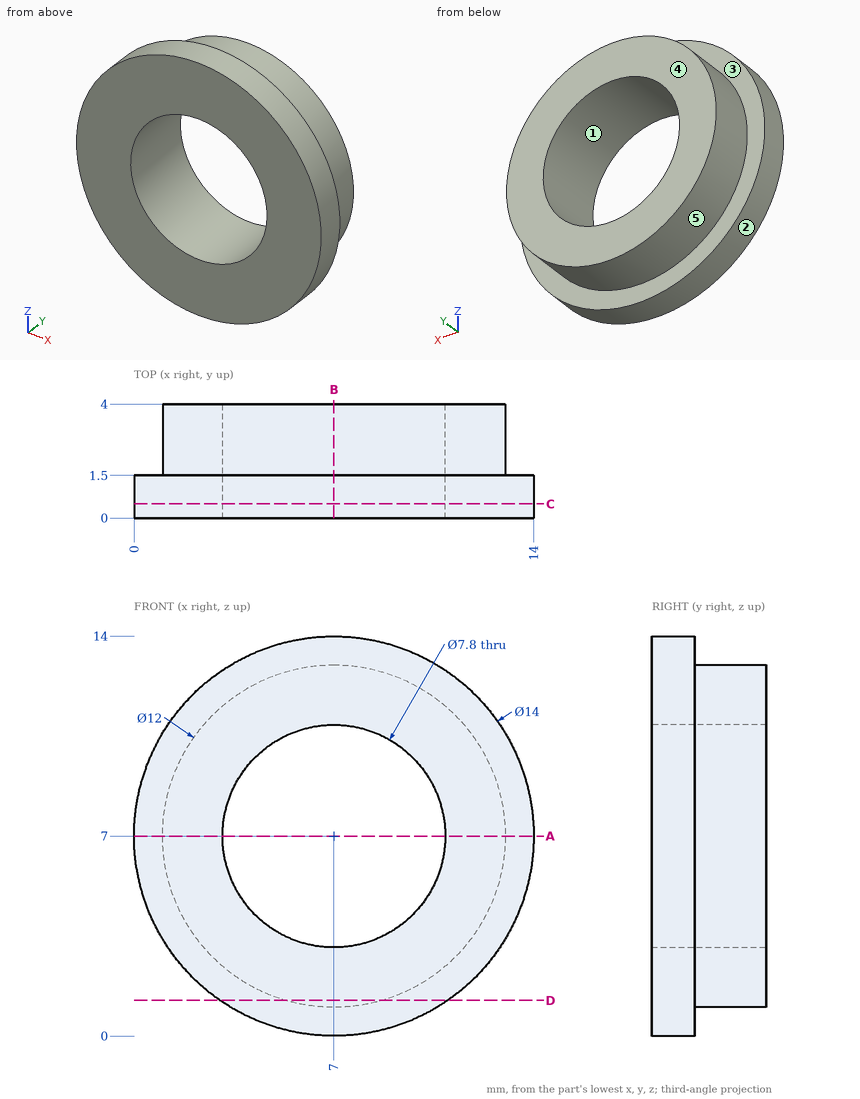
Print and shaded views of the part. All mm, measured from the part's lowest x, y and z. A direction names the side the tool comes from. Round coordinates to 2 decimals unless told otherwise and drop trailing zeros. Write each loop counter-clockwise with the first axis right and the second up, starting at its lowest first coordinate (ties: lowest second). Pieces come first, ordered by that corner, then holes. Notation, with made-up numbers: M -17,-12.75 L 21,-12.75 A26 cw 21,24.25 Z; hole C -6,-34 d8. An arc over 180 degrees is marked long. Use a Markdown table: item, result. Add a question column.
1. Slice it at C-C on y = 0.5. Give the cut face in (x, z).
2. Slice it at B-B on x = 7. Give the cut face in (y, z), then the cut area to 3 significant figures.
3. Slice it at D-D on z = 1.25. Give the cut face in (x, y), then the cut area to 3 significant figures.
4. Pull direction X, two halves, no side cores. Call the marked faces 1, 2 and 3: released by +X, released by -X, zero draft, split by the parting line, or undercut.
5. Flat gauge pins, fed straight in: P1, Ø1.5, axis at x = 3.5, y = 1, coming from the -Z side; P2, Ø1, axis at y = 1.5, z = 2, coming from the -X side. Where does each tip first touch, or does it go through?
6. 3-axis set-ups, long thin cutter, end or side, ignore diameter. For the marked faces 4 and 5: which of +Z, -Z, +X, -X, +Y, -Y reach the whole face in a straight line?
7. Drill centre lines: probe 1 along X at (y, z) = (2.85, 7); probe 2 along X at (y, z) = (0.7, 5); probe 3 along Y at (x, z) = (4, 1.25). Where is each one in solid material? Low to high.
8. Slice it at A-A on z = 7. Give the cut face in (x, y), then the cut area to 3 significant figures.
Reply:
| question | item | result |
|---|---|---|
| 1 | outline | C 7,7 d14; hole C 7,7 d7.8 |
| 2 | outline | M 0,0 L 1.5,0 L 1.5,1 L 4,1 L 4,3.1 L 0,3.1 Z; M 0,10.9 L 4,10.9 L 4,13 L 1.5,13 L 1.5,14 L 0,14 Z |
| 2 | area | 19.8 mm^2 |
| 3 | outline | M 3.01,0 L 10.99,0 L 10.99,1.5 L 8.71,1.5 L 8.71,4 L 5.29,4 L 5.29,1.5 L 3.01,1.5 Z |
| 3 | area | 20.5 mm^2 |
| 4 | face 1 | undercut |
| 4 | face 2 | split by the parting line |
| 4 | face 3 | zero draft |
| 5 | P1 | stops at z = 0.56 |
| 5 | P2 | stops at x = 1.64 |
| 6 | face 4 | +Z, -Z, +X, -X, +Y |
| 6 | face 5 | +Y |
| 7 | probe 1 | x = 1 to 3.1, 10.9 to 13 |
| 7 | probe 2 | x = 0.29 to 3.65, 10.35 to 13.71 |
| 7 | probe 3 | y = 0 to 1.5 |
| 8 | outline | M 0,0 L 3.1,0 L 3.1,4 L 1,4 L 1,1.5 L 0,1.5 Z; M 10.9,0 L 14,0 L 14,1.5 L 13,1.5 L 13,4 L 10.9,4 Z |
| 8 | area | 19.8 mm^2 |
